from build123d import *

# Parameters (mm, degrees)
SKETCH1_W           = 100
SKETCH1_H           = 5
SKETCH1_R           = 1.75
SKETCH1_W_2         = 300
SKETCH1_H_2         = 50
BOSS_EXTRUDE1_DEPTH = 5
SKETCH2_R           = 1.75
CUT_EXTRUDE1_DEPTH  = 10


with BuildPart() as part:
    # Sketch1 → Boss-Extrude1 (new body)
    # profile 1 of 5: a face of its own
    with BuildSketch(Plane(origin=(0, 0, 0), x_dir=(1, 0, 0), z_dir=(0, 1, 0))):
        with Locations((-92.5, -2.5)):
            Rectangle(SKETCH1_W, SKETCH1_H)
        with Locations(Location((-51.75, -2.5, 0), (0, 0, 270))):
            Circle(SKETCH1_R, mode=Mode.SUBTRACT)
        with Locations(Location((-133.25, -2.5, 0), (0, 0, 270))):
            Circle(SKETCH1_R, mode=Mode.SUBTRACT)
    # profile 2 of 5: a face of its own
    with BuildSketch(Plane(origin=(0, 0, 0), x_dir=(1, 0, 0), z_dir=(0, 1, 0))):
        with Locations((0, 25)):
            Rectangle(SKETCH1_W_2, SKETCH1_H_2)
    # profile 3 of 5: a face of its own
    with BuildSketch(Plane(origin=(0, 0, 0), x_dir=(1, 0, 0), z_dir=(0, 1, 0))):
        with Locations((92.5, -2.5)):
            Rectangle(SKETCH1_W, SKETCH1_H)
        with Locations(Location((51.75, -2.5, 0), (0, 0, 270))):
            Circle(SKETCH1_R, mode=Mode.SUBTRACT)
        with Locations(Location((133.25, -2.5, 0), (0, 0, 270))):
            Circle(SKETCH1_R, mode=Mode.SUBTRACT)
    # profile 4 of 5: a face of its own
    with BuildSketch(Plane(origin=(0, 0, 0), x_dir=(1, 0, 0), z_dir=(0, 1, 0))):
        with Locations((92.5, 52.5)):
            Rectangle(SKETCH1_W, SKETCH1_H)
        with Locations(Location((133.25, 52.5, 0), (0, 0, 90))):
            Circle(SKETCH1_R, mode=Mode.SUBTRACT)
        with Locations(Location((51.75, 52.5, 0), (0, 0, 270))):
            Circle(SKETCH1_R, mode=Mode.SUBTRACT)
    # profile 5 of 5: a face of its own
    with BuildSketch(Plane(origin=(0, 0, 0), x_dir=(1, 0, 0), z_dir=(0, 1, 0))):
        with Locations((-92.5, 52.5)):
            Rectangle(SKETCH1_W, SKETCH1_H)
        with Locations(Location((-51.75, 52.5, 0), (0, 0, 90))):
            Circle(SKETCH1_R, mode=Mode.SUBTRACT)
        with Locations(Location((-133.25, 52.5, 0), (0, 0, 270))):
            Circle(SKETCH1_R, mode=Mode.SUBTRACT)
    extrude(amount=BOSS_EXTRUDE1_DEPTH)

    # Sketch2 → Cut-Extrude1 (cut)
    with BuildSketch(Plane(origin=(0, 5, 0), x_dir=(1, 0, 0), z_dir=(0, 1, 0))):
        with Locations(Location((-145, 25, 0), (0, 0, 270))):
            Circle(SKETCH2_R)
        with Locations(Location((145, 25, 0), (0, 0, 270))):
            Circle(SKETCH2_R)
    extrude(amount=-CUT_EXTRUDE1_DEPTH, mode=Mode.SUBTRACT)


solid = part.part
Input: part model. Units: mm. Frame: model coordinates. A direction names the side the tool comes from. Coordinates: 2 decimals unless noted, no trailing zeros. Loops run counter-clockwise (first coordinate to the right, second up) from the corner with the lowest first, then second, coordinate; pieces in that order, holes last. Notation, with made-up numbers: (-30.5, 6) -> (-17.5, 6) arc R23 ccw to (-17.5, 43) -> close; hole circle Ø11 at (50.5, 73.25). An arc over 180 degrees is marked (long way). Write each question's results on one line, items separated by ' | '. Start each with the question number.
Q1. Reachability of faces 1 (the flat face through (-42.5, 2, -52)), 2 (the flat face through (146, 2, 0)), 3 (the flat face through (-42.5, 2, 3)) from +Z, -Z, +X, -X, +Y, -Y: full face, straight path, thin tool, end or side. Return the list, or none.
Q2. Section B-B, the plane x = 9.5. Return the cut outline in (y, z).
Q3. Pin query (flat end, axial travel): pin 1 (1.5 mm diameter, centred on y = 3.5, z = 2.5, fed in from -X); pin 2 (2.5 mm diameter, centred on y = 2, z = 2.5, fed in from +X); pin 3 (2.5 mm diameter, centred on x = 20.5, y = 3.5, fed in from +Z). Return the tip coordinate at first contact, or that it passes through.
Q4. Ray query, line 1 (X direction, y = 1.6, z = -52.5); line 2 (X direction, y = 2.95, z = -50.5); line 3 (Z direction, x = 145, y = 1.6). Return the intervals inside material, ascending. Write a range as from..to.
Q5. Section A-A, the plane y = 2.45. State how many separate pieces and enclosed holes the cut face has, plus the area to 3 significant figures.
Found:
1) face 1: -Z, +Y, -Y | face 2: +Z, +X, +Y, -Y | face 3: +Z, +Y, -Y
2) outline: (0, -50) -> (5, -50) -> (5, 0) -> (0, 0) -> close
3) pin 1: x = -142.5 | pin 2: x = 142.5 | pin 3: z = 0
4) line 1: -142.5..-135, -131.5..-53.5, -50..-42.5, 42.5..50, 53.5..131.5, 135..142.5 | line 2: -142.5..-42.5, 42.5..142.5 | line 3: -50..-26.75, -23.25..0
5) separate pieces: 1 | enclosed holes: 10 | area: 16,900 mm2
